```python
from build123d import *

# Parameters (mm, degrees)
SKETCH_1_W      = 159
SKETCH_1_H      = 159
EXTRUDE_1_DEPTH = 20
CHAMFER_1_SIZE  = 20


with BuildPart() as part:
    # 草图1 → 凸台-拉伸1 (new body)
    with BuildSketch(Plane.XY):
        Rectangle(SKETCH_1_W, SKETCH_1_H)
    extrude(amount=EXTRUDE_1_DEPTH)

    # 倒角1
    chamfer_1_edges = [part.edges().sort_by_distance(p)[0] for p in [
        (79.5, -79.5, 10),
        (-79.5, -79.5, 10),
        (-79.5, 79.5, 10),
        (79.5, 79.5, 10),
    ]]
    chamfer(chamfer_1_edges, length=CHAMFER_1_SIZE)


solid = part.part
```
Input: part model. Units: mm. Frame: model coordinates. Round coordinates to 2 decimals unless told otherwise and drop trailing zeros. Order: outer loops, then holes, each group sorted by start corner. A loop starts at its lowest first (then second) coordinate and runs counter-clockwise, first axis right, second up. Notation, with made-up numbers: (35, 86) - (71, 86) arc R12 cw to (71, 99) - close; hole circle Ø7 at (16, 69.25). An arc over 180 degrees is marked (long way). Answer in a Markdown table with one row per item.
Item 1: Section query B-B (y = -67.5). Return the cut outline in (x, z).
Model answer:
| item | result |
|---|---|
| outline | (-71.5, 0) - (71.5, 0) - (71.5, 20) - (-71.5, 20) - close |
Item 2: Section query A-A (z = 16.75). Return the cut outline in (x, y), then the cut area to 3 significant figures.
Model answer:
| item | result |
|---|---|
| outline | (-79.5, -59.5) - (-59.5, -79.5) - (59.5, -79.5) - (79.5, -59.5) - (79.5, 59.5) - (59.5, 79.5) - (-59.5, 79.5) - (-79.5, 59.5) - close |
| area | 24,500 mm² |
Item 3: Line query: line 1 (Y direction, x = 73, z = 10); line 2 (Y direction, x = 73.5, z = 11); line 3 (X direction, y = -61, z = 12). Output: solid intervals per line, ascending.
Model answer:
| item | result |
|---|---|
| line 1 | y = -66 to 66 |
| line 2 | y = -65.5 to 65.5 |
| line 3 | x = -78 to 78 |
